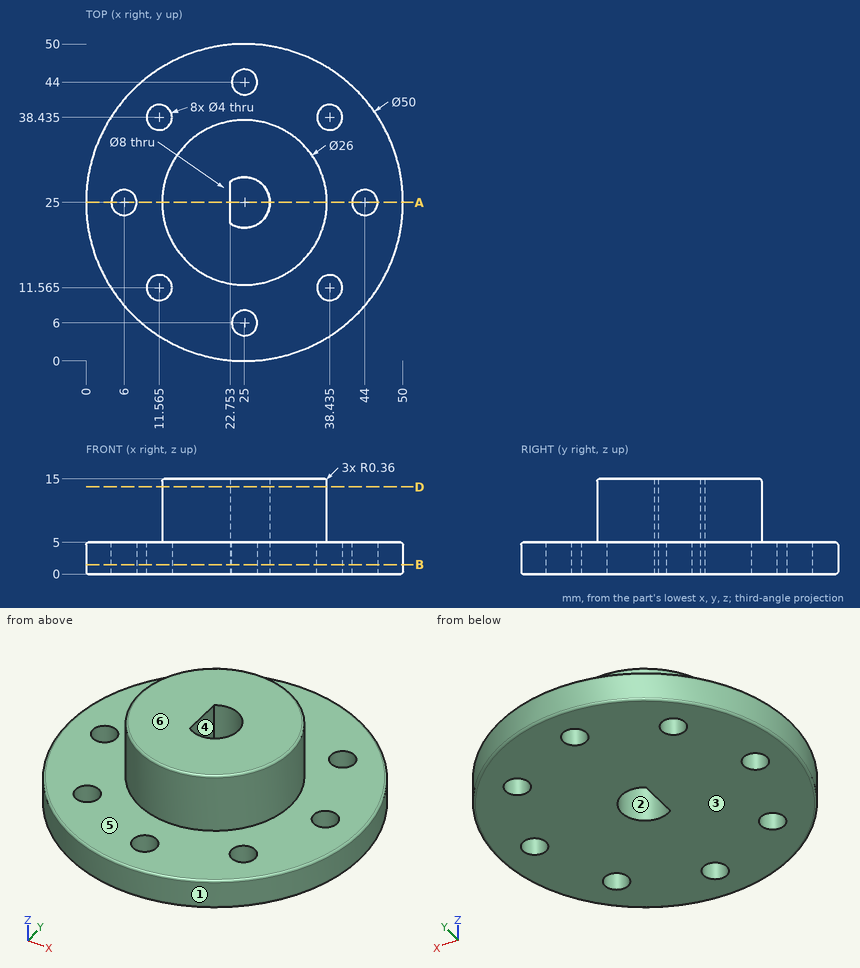
Here's the drawing with two shaded views (mm, measured from the low corner). I have some questions. A direction names the side the tool comes from. Coordinates: 2 decimals unless noted, no trailing zeros. Loops run counter-clockwise (first coordinate to the right, second up) from the corner with the lowest first, then second, coordinate; pieces in that order, holes last. Notation, with made-up numbers: (-4.5, -25.5) -> (10.5, -25.5) arc R31 ccw to (10.5, 1.5) -> close; hole circle Ø4 at (15, 83.5). An arc over 180 degrees is marked (long way). Answer as a JSON object with one key per item and string values.
1) If I drill on line 1 (Y direction, x = 25, z = 3.95); line 2 (X direction, y = 13, z = 4.5); line 3 (Y direction, x = 38.5, z = 2.75) (1 decimal), over which ranges is the centre line in solid material (lowest first)?
Results:
{"line 1": "y = 0 to 4, 8 to 21, 29 to 42, 46 to 50", "line 2": "x = 3.07 to 10.17, 12.96 to 37.04, 39.83 to 46.93", "line 3": "y = 4 to 9.6, 13.6 to 36.4, 40.4 to 46"}
2) Imagine slicing it at D-D (z = 13.75). Please give me the cut outline in (x, y).
Results:
{"outline": "circle Ø26 at (25, 25); hole (22.75, 21.69) arc R4 ccw (long way) to (22.75, 28.31) -> close"}
3) Imagine slicing it at A-A (y = 25). Please give me the cut outline in (x, z).
Results:
{"outline": "(0, 0.36) arc R0.36 ccw to (0.36, 0) -> (4, 0) -> (4, 5) -> (0.36, 5) arc R0.36 ccw to (0, 4.64) -> close; (8, 0) -> (22.75, 0) -> (22.75, 15) -> (12.36, 15) arc R0.36 ccw to (12, 14.64) -> (12, 5) -> (8, 5) -> close; (29, 0) -> (42, 0) -> (42, 5) -> (38, 5) -> (38, 14.64) arc R0.36 ccw to (37.64, 15) -> (29, 15) -> close; (46, 0) -> (49.64, 0) arc R0.36 ccw to (50, 0.36) -> (50, 4.64) arc R0.36 ccw to (49.64, 5) -> (46, 5) -> close"}
4) Thinking about a two-plate mould opening in Y: for the marked faces 1, 2 and 3, which applies, pulls with the +Y half, pulls with the -Y half, needs draft (parallel to the pull), parting line crosses it, or undercut?
Results:
{"face 1": "parting line crosses it", "face 2": "undercut", "face 3": "needs draft"}
5) For P1, Ø1, axis at y = 21, z = 4, coming from the -X side; P2, Ø8, axis at y = 25.5, z = 10.5, coming from the +X side; P3, Ø6.5, axis at x = 38.44, y = 11.56, coming from the +Z side; P4, Ø2.5, axis at x = 25, y = 44, coming from the +Z side, each with a flat end and sliding along its axis, tell me the tip position at first contact or that it passes through.
Results:
{"P1": "stops at x = 0.25", "P2": "stops at x = 38", "P3": "stops at z = 5", "P4": "passes through"}
6) Imagine slicing it at B-B (z = 1.5). Count the separate pieces of the cut face and the enclosed holes in it, then the cut area to 3 significant figures.
Results:
{"separate pieces": "1", "enclosed holes": "9", "area": "1,820 mm^2"}
7) For the marked faces 4, 5 and 6, which set-ups out of +Z, -Z, +X, -X, +Y, -Y let a thin tool reach every point of the face, with its end or its side?
Results:
{"face 4": "+Z, -Z", "face 5": "+Z", "face 6": "+Z, +X, -X, +Y, -Y"}
